Work out the finished part from the listing and answer in its coordinate system (mm). Give positions to 0.01 mm unless a question says otherwise; leave off trailing zeros. Write each loop counter-clockwise with the first axis right and the second up, starting at its lowest first coordinate (ties: lowest second). Pieces come first, ordered by that corner, then holes. Notation, with made-up numbers: (68.25, -13) - (82.25, -13) arc R20 cw to (82.25, 20) - close; hole circle Ø8 at (-35, -25). An arc over 180 degrees is marked (long way). Write item = value, one per line.
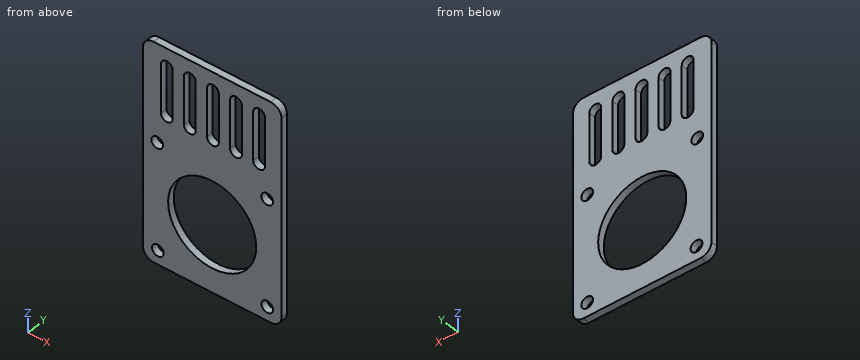
from build123d import *

# Parameters (mm, degrees)
SKETCH_1_R      = 2.55
SKETCH_1_R_2    = 19.1
EXTRUDE_1_DEPTH = 3


with BuildPart() as part:
    # Эскиз1 → Бобышка-Вытянуть1 (new body)
    with BuildSketch(Plane(origin=(0, 0, 0), x_dir=(1, 0, 0), z_dir=(0, 1, 0))):
        with BuildLine():
            Line((4.6, 0), (55.4, 0))
            ThreePointArc((55.4, 0), (58.652691193, -1.347308807), (60, -4.6))
            Line((60, -4.6), (60, -91.9))
            ThreePointArc((60, -91.9), (58.652691193, -95.152691193), (55.4, -96.5))
            Line((55.4, -96.5), (4.6, -96.5))
            ThreePointArc((4.6, -96.5), (1.347308807, -95.152691193), (0, -91.9))
            Line((0, -91.9), (0, -4.6))
            ThreePointArc((0, -4.6), (1.347308807, -1.347308807), (4.6, 0))
        make_face()
        with Locations(Location((6.45, -6.15, 0), (0, 0, 270))):
            Circle(SKETCH_1_R, mode=Mode.SUBTRACT)
        with Locations(Location((53.85, -6.15, 0), (0, 0, 270))):
            Circle(SKETCH_1_R, mode=Mode.SUBTRACT)
        with Locations(Location((6.15, -53.25, 0), (0, 0, 270))):
            Circle(SKETCH_1_R, mode=Mode.SUBTRACT)
        with Locations(Location((53.85, -53.25, 0), (0, 0, 270))):
            Circle(SKETCH_1_R, mode=Mode.SUBTRACT)
        with Locations(Location((30, -29.7, 0), (0, 0, 270))):
            Circle(SKETCH_1_R_2, mode=Mode.SUBTRACT)
        with BuildLine():
            Line((12.861404853, -66.95), (12.861404853, -88.45))
            ThreePointArc((12.861404853, -88.45), (10.311404853, -91), (7.761404853, -88.45))
            Line((7.761404853, -88.45), (7.761404853, -66.95))
            ThreePointArc((7.761404853, -66.95), (10.311404853, -64.4), (12.861404853, -66.95))
        make_face(mode=Mode.SUBTRACT)
        with BuildLine():
            Line((22.861404853, -66.95), (22.861404853, -88.45))
            ThreePointArc((22.861404853, -88.45), (20.311404853, -91), (17.761404853, -88.45))
            Line((17.761404853, -88.45), (17.761404853, -66.95))
            ThreePointArc((17.761404853, -66.95), (20.311404853, -64.4), (22.861404853, -66.95))
        make_face(mode=Mode.SUBTRACT)
        with BuildLine():
            Line((32.861404853, -66.95), (32.861404853, -88.45))
            ThreePointArc((32.861404853, -88.45), (30.311404853, -91), (27.761404853, -88.45))
            Line((27.761404853, -88.45), (27.761404853, -66.95))
            ThreePointArc((27.761404853, -66.95), (30.311404853, -64.4), (32.861404853, -66.95))
        make_face(mode=Mode.SUBTRACT)
        with BuildLine():
            Line((42.861404853, -66.95), (42.861404853, -88.45))
            ThreePointArc((42.861404853, -88.45), (40.311404853, -91), (37.761404853, -88.45))
            Line((37.761404853, -88.45), (37.761404853, -66.95))
            ThreePointArc((37.761404853, -66.95), (40.311404853, -64.4), (42.861404853, -66.95))
        make_face(mode=Mode.SUBTRACT)
        with BuildLine():
            Line((52.861404853, -66.95), (52.861404853, -88.45))
            ThreePointArc((52.861404853, -88.45), (50.311404853, -91), (47.761404853, -88.45))
            Line((47.761404853, -88.45), (47.761404853, -66.95))
            ThreePointArc((47.761404853, -66.95), (50.311404853, -64.4), (52.861404853, -66.95))
        make_face(mode=Mode.SUBTRACT)
    extrude(amount=EXTRUDE_1_DEPTH)


solid = part.part
1. Given pin 1 (6 mm diameter, centred on x = 6, z = 69, fed in from -Y); pin 2 (3 mm diameter, centred on x = 47, z = 31, fed in from -Y), each flat-ended and moving along its own axis, determine where each tip first touches the part or whether it passes through.
Solution:
pin_1 = 0
pin_2 = through
2. Straight lines are drawn through the part: line 1 (X direction, y = 2.05, z = 6.15); line 2 (X direction, y = 2.3, z = 87); line 3 (Z direction, x = 39, y = 0.7). For each, find the intervals that lie inside material, in ascending order.
Solution:
line_1 = 0 to 3.9, 9 to 51.3, 56.4 to 60
line_2 = 0 to 7.76, 12.86 to 17.76, 22.86 to 27.76, 32.86 to 37.76, 42.86 to 47.76, 52.86 to 60
line_3 = 0 to 12.85, 46.55 to 64.76, 90.64 to 96.5
3. Find section D-D, the plane z = 29.7. Give the vertices of the cut face in (x, y).
Solution:
outline = (0, 0) - (10.9, 0) - (10.9, 3) - (0, 3) - close; (49.1, 0) - (60, 0) - (60, 3) - (49.1, 3) - close
4. Find section A-A, the plane z = 6.15. Give the vertices of the cut face in (x, y), then the cut area to 3 significant figures.
Solution:
outline = (0, 0) - (3.9, 0) - (3.9, 3) - (0, 3) - close; (9, 0) - (51.3, 0) - (51.3, 3) - (9, 3) - close; (56.4, 0) - (60, 0) - (60, 3) - (56.4, 3) - close
area = 149 mm^2
5. Find section C-C, the plane y = 1.2. Give the number of separate pieces and of enclosed holes in the cut face, then the cut area to 3 significant figures.
Solution:
separate_pieces = 1
enclosed_holes = 10
area = 3,890 mm^2
6. Find section B-B, the plane z = 76.5. Give the vertices of the cut face in (x, y).
Solution:
outline = (0, 0) - (7.76, 0) - (7.76, 3) - (0, 3) - close; (12.86, 0) - (17.76, 0) - (17.76, 3) - (12.86, 3) - close; (22.86, 0) - (27.76, 0) - (27.76, 3) - (22.86, 3) - close; (32.86, 0) - (37.76, 0) - (37.76, 3) - (32.86, 3) - close; (42.86, 0) - (47.76, 0) - (47.76, 3) - (42.86, 3) - close; (52.86, 0) - (60, 0) - (60, 3) - (52.86, 3) - close
